CAD build for the part. Positions are in the model's coordinates, mm. Face numbers are marked on the shaded views. Coordinates: 2 decimals unless noted, no trailing zeros. Loops run counter-clockwise (first coordinate to the right, second up) from the corner with the lowest first, then second, coordinate; pieces in that order, holes last. Notation, with made-up numbers: (1, -35) - (23, -35) arc R20 ccw to (23, -30) - close; hole circle Ø5 at (-14.5, -21). An arc over 180 degrees is marked (long way). Put each result on its own line as item: value.
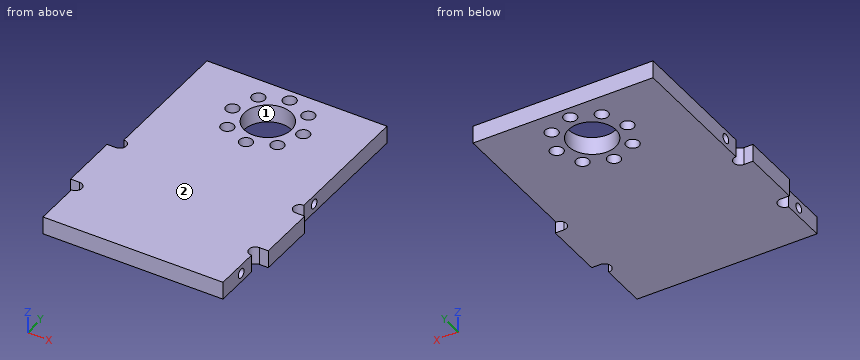
Autodesk Inventor part; units mm, degrees
ref_plane "YZ Plane" through (0, 0, 0) normal (1, 0, 0) x (0, 1, 0)
ref_plane "XZ Plane" through (0, 0, 0) normal (0, 1, 0) x (-1, 0, 0)
ref_plane "XY Plane" through (0, 0, 0) normal (0, 0, 1) x (1, 0, 0)
sketch "スケッチ1" plane through (0, 0, 0) normal (0, 0, 1) x (1, 0, 0)
  line L0 (-15.25, -22.5) -> (15.25, -22.5)
  line L1 (15.25, -22.5) -> (15.25, 22.5)
  line L2 (15.25, 22.5) -> (-15.25, 22.5)
  line L3 (-15.25, 22.5) -> (-15.25, -22.5)
  line L4 (-15.25, -22.5) -> (15.25, 22.5) construction
  line L5 (15.25, -22.5) -> (-15.25, 22.5) construction
  point P0 (0, 0)
  dimension "d0" = 30.5
  dimension "d1" = 45
extrude "押し出し1" add sketch "スケッチ1" along normal blind 3
sketch "スケッチ2" plane through (0, 0, 3) normal (0, 0, 1) x (1, 0, 0)
  line L0 (-15.25, -2.5) -> (-16.75, -2.5)
  line L1 (-16.75, -2.5) -> (-16.75, -12.5)
  line L2 (-16.75, -12.5) -> (-15.25, -12.5)
  line L3 (-15.25, -12.5) -> (-15.25, -2.5)
  line L4 (-15.25, 22.5) -> (-15.25, -22.5)
  line L5 (-15.25, -22.5) -> (15.25, -22.5)
  circle A0 centre (-15.25, -13.6) radius 1.1
  circle A1 centre (-15.25, -1.4) radius 1.1
  line L6 (15.25, 22.5) -> (-15.25, 22.5) construction
  line L7 (0, 22.5) -> (0, 0) construction
  line L8 (15.25, -2.5) -> (16.75, -2.5)
  line L9 (16.75, -2.5) -> (16.75, -12.5)
  line L10 (16.75, -12.5) -> (15.25, -12.5)
  line L11 (15.25, -12.5) -> (15.25, -2.5)
  circle A2 centre (15.25, -13.6) radius 1.1
  circle A3 centre (15.25, -1.4) radius 1.1
  point P0 (-15.25, -0.3)
  point P1 (-15.25, -14.7)
  dimension "d7" = 2.2
  dimension "d4" = 10
  dimension "d5" = 1.5
  dimension "d6" = 10
extrude "押し出し2" add sketch "スケッチ2" against normal up to surface (3 mm away) contours L3 L2 L1 L0 | L8 L9 L10 L11
extrude "押し出し3" cut sketch "スケッチ2" against normal through all contours A0 L4 | L4 A1 | A2 | A3 picked at (-14.7226, -13.8557) picked at (-14.9196, -1.2409)
sketch "スケッチ3" plane through (-15.25, 22.5, 0) normal (-1, 0, 0) x (0, 0, 1)
  line L0 (3, -25) -> (0, -25)
  line L1 (3, -35) -> (0, -35)
  point P0 (0, -22.5)
  point P1 (1.5, -20)
  point P2 (1.5, -40)
  point P3 (1.5, -25)
  point P4 (1.5, -35)
  point P5 (1.5, -25)
  point P6 (1.5, -35)
  dimension "d12" = 5
  dimension "d13" = 5
hole "穴1" at (-15.25, 2.5, 1.5) at (-15.25, -17.5, 1.5) direction (1, 0, 0) diameter 1.567 end through all
sketch "スケッチ4" plane through (0, 0, 3) normal (0, 0, 1) x (1, 0, 0)
  circle A0 centre (0, 14.5) radius 8
  line L0 (15.25, 22.5) -> (-15.25, 22.5)
  circle A1 centre (0, 14.5) radius 4
  circle A2 centre (0, 14.5) radius 6 construction
  circle A3 centre (0, 8.5) radius 1.1
  circle A4 centre (4.2426, 10.2574) radius 1.1
  circle A5 centre (6, 14.5) radius 1.1
  circle A6 centre (4.2426, 18.7426) radius 1.1
  circle A7 centre (0, 20.5) radius 1.1
  circle A8 centre (-4.2426, 18.7426) radius 1.1
  circle A9 centre (-6, 14.5) radius 1.1
  circle A10 centre (-4.2426, 10.2574) radius 1.1
  point P0 (0, 0)
  point P1 (0, 22.5)
  dimension "d23" = 12
  dimension "d21" = 16
  dimension "d22" = 8
  dimension "d24" = 2.2
  dimension "d27" = 360
extrude "押し出し4" cut sketch "スケッチ4" against normal through all contours A1 | A3 | A4 | A5 | A6 | A7 | A8 | A9 | A10
properties part number "kosiyo"
Q1. Slice it at C-C, the plane z = 1.5. State how many separate pieces and enclosed holes the cut face has, then the cut area to 3 significant figures.
Determined:
separate pieces: 3
enclosed holes: 9
area: 1,220 mm2
Q2. Pin check, flat tips, straight feed: pin 1 Ø1.5 at (y, z) = (17, 1) entering from -X; pin 2 Ø1.5 at (y, z) = (-17.5, 2) entering from +X; pin 3 Ø0.8 at (x, z) = (16.5, 1.5) entering from +Y. Stop position of each tip, or through.
Determined:
pin 1: x = -15.25
pin 2: x = 15.25
pin 3: y = -2.5
Q3. Slice it at B-B, the plane y = -17.5. Give the cut face in (x, z), then the cut area to 3 significant figures.
Determined:
outline: (-15.25, 0) - (15.25, 0) - (15.25, 0.72) - (-15.25, 0.72) - close; (-15.25, 2.28) - (15.25, 2.28) - (15.25, 3) - (-15.25, 3) - close
area: 43.7 mm2
Q4. Wall check: L1, parallel to Y at x = 6, z = 1.6; L2, parallel to Y at x = 5, z = 2.4; L3, parallel to X at y = -16, z = 0.85. Give the ranges that are in metal, low to high. Write a range as from..to.
Determined:
L1: -22.5..-18.28, -16.72..1.72, 3.28..13.4, 15.6..22.5
L2: -22.5..9.46, 11.06..14.04, 14.96..17.94, 19.54..22.5
L3: -15.25..15.25
Q5. Mould opens along Y. For the marked faces 1 and 2 say: +Y half, -Y half, draft (parallel to the pull), parting line (faces both ways), or undercut.
Determined:
face 1: undercut
face 2: draft
Q6. Slice it at A-A, the plane x = 6. Give the cut face in (y, z).
Determined:
outline: (-22.5, 0) - (13.4, 0) - (13.4, 3) - (-22.5, 3) - close; (15.6, 0) - (22.5, 0) - (22.5, 3) - (15.6, 3) - close; hole circle Ø1.57 at (-17.5, 1.5); hole circle Ø1.57 at (2.5, 1.5)
Q7. Slice it at D-D, the plane y = 8.5. Give the cut face in (x, z).
Determined:
outline: (-15.25, 0) - (-1.1, 0) - (-1.1, 3) - (-15.25, 3) - close; (1.1, 0) - (15.25, 0) - (15.25, 3) - (1.1, 3) - close
